```python
from build123d import *

# Parameters (mm, degrees)
SKETCH_1_R          = 30
EXTRUDE_1_DEPTH     = 21
SKETCH_2_R          = 21
CUT_EXTRUDE_1_DEPTH = 17
SKETCH_4_R          = 1.55
SKETCH_4_R_2        = 4.384489401
CUT_EXTRUDE_3_DEPTH = 17


with BuildPart() as part:
    # 草图1 → 凸台-拉伸1 (new body)
    with BuildSketch(Plane(origin=(0, 0, 0), x_dir=(1, 0, 0), z_dir=(0, 1, 0))):
        with Locations(Location((0, 0, 0), (0, 0, 90))):
            Circle(SKETCH_1_R)
    extrude(amount=EXTRUDE_1_DEPTH)

    # 草图2 → 切除-拉伸1 (cut)
    with BuildSketch(Plane.XZ):
        with Locations(Location((0, 0, 0), (0, 0, 270))):
            Circle(SKETCH_2_R)
    extrude(amount=-CUT_EXTRUDE_1_DEPTH, mode=Mode.SUBTRACT)

    # 草图4 → 切除-拉伸3 (cut)
    with BuildSketch(Plane(origin=(0, 21, 0), x_dir=(1, 0, 0), z_dir=(0, 1, 0))):
        with Locations(Location((-6, 0, 0), (0, 0, 270))):
            Circle(SKETCH_4_R)
        with Locations(Location((0, 6.5, 0), (0, 0, 270))):
            Circle(SKETCH_4_R)
        with Locations(Location((6, 0, 0), (0, 0, 270))):
            Circle(SKETCH_4_R)
        with Locations(Location((0, -6.5, 0), (0, 0, 270))):
            Circle(SKETCH_4_R)
        with Locations(Location((0, 0, 0), (0, 0, 270))):
            Circle(SKETCH_4_R_2)
        with BuildLine():
            ThreePointArc((11.79815708, 14.077346516), (0.167157726, 18.366824813), (-11.539986211, 14.289748551))
            ThreePointArc((-11.539986211, 14.289748551), (-11.796674112, 11.878565481), (-9.385491043, 11.62187758))
            ThreePointArc((-9.385491043, 11.62187758), (0.135949672, 14.93777086), (9.595461863, 11.449130632))
            ThreePointArc((9.595461863, 11.449130632), (12.010917413, 11.661890965), (11.79815708, 14.077346516))
        make_face()
        with BuildLine():
            ThreePointArc((11.79815708, -14.077346516), (0.167157726, -18.366824813), (-11.539986211, -14.289748551))
            ThreePointArc((-11.539986211, -14.289748551), (-11.796674112, -11.878565481), (-9.385491043, -11.62187758))
            ThreePointArc((-9.385491043, -11.62187758), (0.135949672, -14.93777086), (9.595461863, -11.449130632))
            ThreePointArc((9.595461863, -11.449130632), (12.010917413, -11.661890965), (11.79815708, -14.077346516))
        make_face()
    extrude(amount=-CUT_EXTRUDE_3_DEPTH, mode=Mode.SUBTRACT)


solid = part.part
```
Geometry check sheet. Reference: the model listing, model coordinates, mm. A direction names the side the tool comes from. Coordinates: 2 decimals unless noted, no trailing zeros. Loops run counter-clockwise (first coordinate to the right, second up) from the corner with the lowest first, then second, coordinate; pieces in that order, holes last. Notation, with made-up numbers: (-21, -24) - (33, -24) arc R13 ccw to (33, 1) - close; hole circle Ø3 at (19.5, 64.5). An arc over 180 degrees is marked (long way). One line per item, written item: value. Start each with the question number.
(1) Cross-section at D-D on x = 6. Enter the section's corners in (y, z), plus the area to 3 significant figures.
(2) Cross-section at B-B on z = 0. Enter the section's corners in (x, y).
(3) Tool access check on faces 4 (the flat face through (6, 21, -6)), 5 (the cylindrical face through (0.344, 19.028, -18.364)), 6 (the cylindrical face through (6.31, 8.38, -20.03)). Record the directions out of +Z, -Z, +X, -X, +Y, -Y that give a thin tool (end or side, any length) a straight path to the whole face; none if there is none.
(4) Cross-section at A-A on x = 0. Enter the section's corners in (y, z).
(5) Mould release check, pull along Z, two halves, no side actions. Record for faces 1 (the flat face through (-20.4, 0, -6.2)), 2 (the cylindrical face through (11.986, 19.028, -11.633)), 3 (the cylindrical face through (-1.32, 10.35, 29.97)): released by +Z, released by -Z, zero draft, split by the parting line, or undercut.
(6) Material ranges on line 1 (X direction, y = 8.25, z = 0); line 2 (Z direction, x = 17.5, y = 11); line 3 (Z direction, x = 18, y = 15), recorded low to high. Write a range as [from, to].
(7) Cross-section at C-C on y = 6. Enter the section's corners in (x, z).
(8) Depth check by flat-ended pin: P1, Ø6, axis at y = 9, z = -7.5, coming from the -X side; P2, Ø5, axis at x = 5, y = 17, coming from the -Z side; P3, Ø1.9, axis at x = 0, z = -6.5, coming from the +Y side; P4, Ø1.5, axis at y = 8.5, z = 1, coming from the -X side. Enter the tip coordinate at first touch or a pass-through.
Results below:
1. outline: (0, -29.39) - (21, -29.39) - (21, -17.36) - (17, -17.36) - (17, -20.12) - (0, -20.12) - close; (0, 20.12) - (17, 20.12) - (17, 17.36) - (21, 17.36) - (21, 29.39) - (0, 29.39) - close; (17, -13.68) - (21, -13.68) - (21, -1.55) - (17, -1.55) - close; (17, 1.55) - (21, 1.55) - (21, 13.68) - (17, 13.68) - close
1. area: 508 mm2
2. outline: (-30, 0) - (-21, 0) - (-21, 17) - (-7.55, 17) - (-7.55, 21) - (-30, 21) - close; (-4.45, 17) - (-4.38, 17) - (-4.38, 21) - (-4.45, 21) - close; (4.38, 17) - (4.45, 17) - (4.45, 21) - (4.38, 21) - close; (7.55, 17) - (21, 17) - (21, 0) - (30, 0) - (30, 21) - (7.55, 21) - close
3. face 4: +Z, -Z, +X, -X, +Y
3. face 5: +Y, -Y
3. face 6: -Y
4. outline: (0, -30) - (21, -30) - (21, -18.37) - (17, -18.37) - (17, -21) - (0, -21) - close; (0, 21) - (17, 21) - (17, 18.37) - (21, 18.37) - (21, 30) - (0, 30) - close; (17, -14.94) - (21, -14.94) - (21, -8.05) - (17, -8.05) - close; (17, -4.95) - (21, -4.95) - (21, -4.38) - (17, -4.38) - close; (17, 4.38) - (21, 4.38) - (21, 4.95) - (17, 4.95) - close; (17, 8.05) - (21, 8.05) - (21, 14.94) - (17, 14.94) - close
5. face 1: zero draft
5. face 2: undercut
5. face 3: split by the parting line
6. line 1: x = [-30, -21], [21, 30]
6. line 2: z = [-24.37, -11.61], [11.61, 24.37]
6. line 3: z = [-24, -10.82], [10.82, 24]
7. outline: circle Ø60 at (0, 0); hole circle Ø42 at (0, 0)
8. P1: stops at x = -29.66
8. P2: stops at z = -29.9
8. P3: passes through
8. P4: stops at x = -30
